```python
from build123d import *

# Parameters (mm, degrees)
EKSTR_ZYON_NCE1_DEPTH = 60
RADYUS1_R             = 10
KES_EKSTR_ZYON1_REACH = 236.137
IZIM2_R               = 4
IZIM2_R_2             = 2
KES_EKSTR_ZYON2_REACH = 234.491
IZIM3_R               = 2.5


with BuildPart() as part:
    # izim1 → Ekstr_zyon-_nce1 (new body)
    with BuildSketch(Plane.XY):
        Polygon((0, 0), (200, 0), (200, 90), (0, 90), (0, 94), (204, 94), (204, -4), (0, -4), align=None)
    extrude(amount=EKSTR_ZYON_NCE1_DEPTH)

    # Radyus1
    radyus1_edges = [part.edges().sort_by_distance(p)[0] for p in [
        (0, -2, 60),
        (0, 92, 60),
        (0, -2, 0),
        (0, 92, 0),
    ]]
    fillet(radyus1_edges, radius=RADYUS1_R)

    # izim2 → Kes-Ekstr_zyon1 (cut, up to next)
    with BuildSketch(Plane(origin=(0, 94, 0), x_dir=(1, 0, 0), z_dir=(0, 1, 0)), mode=Mode.PRIVATE) as kes_ekstr_zyon1_sk1:
        with Locations(Location((23, -30, 0), (0, 0, 270))):
            Circle(IZIM2_R)
    kes_ekstr_zyon1_tool1 = extrude(kes_ekstr_zyon1_sk1.sketch, amount=-KES_EKSTR_ZYON1_REACH, mode=Mode.PRIVATE) & part.part
    # izim2 → Kes-Ekstr_zyon1 (cut, up to next)
    with BuildSketch(Plane(origin=(0, 94, 0), x_dir=(1, 0, 0), z_dir=(0, 1, 0)), mode=Mode.PRIVATE) as kes_ekstr_zyon1_sk2:
        with Locations(Location((23, -22, 0), (0, 0, 270))):
            Circle(IZIM2_R_2)
    kes_ekstr_zyon1_tool2 = extrude(kes_ekstr_zyon1_sk2.sketch, amount=-KES_EKSTR_ZYON1_REACH, mode=Mode.PRIVATE) & part.part
    # izim2 → Kes-Ekstr_zyon1 (cut, up to next)
    with BuildSketch(Plane(origin=(0, 94, 0), x_dir=(1, 0, 0), z_dir=(0, 1, 0)), mode=Mode.PRIVATE) as kes_ekstr_zyon1_sk3:
        with Locations(Location((23, -38, 0), (0, 0, 270))):
            Circle(IZIM2_R_2)
    kes_ekstr_zyon1_tool3 = extrude(kes_ekstr_zyon1_sk3.sketch, amount=-KES_EKSTR_ZYON1_REACH, mode=Mode.PRIVATE) & part.part
    # izim2 → Kes-Ekstr_zyon1 (cut, up to next)
    with BuildSketch(Plane(origin=(0, 94, 0), x_dir=(1, 0, 0), z_dir=(0, 1, 0)), mode=Mode.PRIVATE) as kes_ekstr_zyon1_sk4:
        with Locations(Location((31, -30, 0), (0, 0, 270))):
            Circle(IZIM2_R_2)
    kes_ekstr_zyon1_tool4 = extrude(kes_ekstr_zyon1_sk4.sketch, amount=-KES_EKSTR_ZYON1_REACH, mode=Mode.PRIVATE) & part.part
    # izim2 → Kes-Ekstr_zyon1 (cut, up to next)
    with BuildSketch(Plane(origin=(0, 94, 0), x_dir=(1, 0, 0), z_dir=(0, 1, 0)), mode=Mode.PRIVATE) as kes_ekstr_zyon1_sk5:
        with Locations(Location((15, -30, 0), (0, 0, 270))):
            Circle(IZIM2_R_2)
    kes_ekstr_zyon1_tool5 = extrude(kes_ekstr_zyon1_sk5.sketch, amount=-KES_EKSTR_ZYON1_REACH, mode=Mode.PRIVATE) & part.part
    kes_ekstr_zyon1_1 = kes_ekstr_zyon1_tool1.solids().sort_by_distance((23, 94, 30))[0]
    add(kes_ekstr_zyon1_1, mode=Mode.SUBTRACT)
    kes_ekstr_zyon1_2 = kes_ekstr_zyon1_tool2.solids().sort_by_distance((23, 94, 22))[0]
    add(kes_ekstr_zyon1_2, mode=Mode.SUBTRACT)
    kes_ekstr_zyon1_3 = kes_ekstr_zyon1_tool3.solids().sort_by_distance((23, 94, 38))[0]
    add(kes_ekstr_zyon1_3, mode=Mode.SUBTRACT)
    kes_ekstr_zyon1_4 = kes_ekstr_zyon1_tool4.solids().sort_by_distance((31, 94, 30))[0]
    add(kes_ekstr_zyon1_4, mode=Mode.SUBTRACT)
    kes_ekstr_zyon1_5 = kes_ekstr_zyon1_tool5.solids().sort_by_distance((15, 94, 30))[0]
    add(kes_ekstr_zyon1_5, mode=Mode.SUBTRACT)
    kes_ekstr_zyon1 = kes_ekstr_zyon1_1 + kes_ekstr_zyon1_2 + kes_ekstr_zyon1_3 + kes_ekstr_zyon1_4 + kes_ekstr_zyon1_5  # Kes-Ekstr_zyon1 as one shape, for the pattern or mirror that repeats it

    # Aynalama1: Kes-Ekstr_zyon1 across plane
    add(kes_ekstr_zyon1.mirror(Plane.ZX.offset(45)), mode=Mode.SUBTRACT)

    # izim3 → Kes-Ekstr_zyon2 (cut, up to next)
    with BuildSketch(Plane(origin=(204, 0, 0), x_dir=(0, 0, -1), z_dir=(1, 0, 0)), mode=Mode.PRIVATE) as kes_ekstr_zyon2_sk1:
        with Locations((-30, 60)):
            Circle(IZIM3_R)
    kes_ekstr_zyon2_tool1 = extrude(kes_ekstr_zyon2_sk1.sketch, amount=-KES_EKSTR_ZYON2_REACH, mode=Mode.PRIVATE) & part.part
    # izim3 → Kes-Ekstr_zyon2 (cut, up to next)
    with BuildSketch(Plane(origin=(204, 0, 0), x_dir=(0, 0, -1), z_dir=(1, 0, 0)), mode=Mode.PRIVATE) as kes_ekstr_zyon2_sk2:
        with Locations(Location((-30, 30, 0), (0, 0, 180))):
            Circle(IZIM3_R)
    kes_ekstr_zyon2_tool2 = extrude(kes_ekstr_zyon2_sk2.sketch, amount=-KES_EKSTR_ZYON2_REACH, mode=Mode.PRIVATE) & part.part
    # izim3 → Kes-Ekstr_zyon2 (cut, up to next)
    with BuildSketch(Plane(origin=(204, 0, 0), x_dir=(0, 0, -1), z_dir=(1, 0, 0)), mode=Mode.PRIVATE) as kes_ekstr_zyon2_sk3:
        with Locations((-15, 45)):
            Circle(IZIM3_R)
    kes_ekstr_zyon2_tool3 = extrude(kes_ekstr_zyon2_sk3.sketch, amount=-KES_EKSTR_ZYON2_REACH, mode=Mode.PRIVATE) & part.part
    # izim3 → Kes-Ekstr_zyon2 (cut, up to next)
    with BuildSketch(Plane(origin=(204, 0, 0), x_dir=(0, 0, -1), z_dir=(1, 0, 0)), mode=Mode.PRIVATE) as kes_ekstr_zyon2_sk4:
        with Locations(Location((-45, 45, 0), (0, 0, 180))):
            Circle(IZIM3_R)
    kes_ekstr_zyon2_tool4 = extrude(kes_ekstr_zyon2_sk4.sketch, amount=-KES_EKSTR_ZYON2_REACH, mode=Mode.PRIVATE) & part.part
    add(kes_ekstr_zyon2_tool1.solids().sort_by_distance((204, 60, 30))[0], mode=Mode.SUBTRACT)
    add(kes_ekstr_zyon2_tool2.solids().sort_by_distance((204, 30, 30))[0], mode=Mode.SUBTRACT)
    add(kes_ekstr_zyon2_tool3.solids().sort_by_distance((204, 45, 15))[0], mode=Mode.SUBTRACT)
    add(kes_ekstr_zyon2_tool4.solids().sort_by_distance((204, 45, 45))[0], mode=Mode.SUBTRACT)


solid = part.part
```
Here's how the part is built. I have some questions about the finished solid (model axes, mm). A direction names the side the tool comes from. Give positions to 0.01 mm unless a question says otherwise; leave off trailing zeros. Loops run counter-clockwise (first coordinate to the right, second up) from the corner with the lowest first, then second, coordinate; pieces in that order, holes last. Notation, with made-up numbers: M -1,9 L 54,9 A26 ccw 54,39 Z; hole C -2.75,86 d8. An arc over 180 degrees is marked long. Use one line per item in the form item = value. Start each with the question number.
Q1. If we section it at C-C (y = 60): Write out the boundary of the cut face in (x, z).
Q2. I need wall thicknesses on line 1 along X through (y, z) = (91, 30); line 2 along Y through (x, z) = (176, 20); line 3 along Z through (x, y) = (201, 30). Which ranges of each line are inside material? Lowest first, please.
Q3. If we section it at D-D (x = 15): Write out the boundary of the cut face in (y, z).
Q4. If we section it at A-A (x = 147): Write out the boundary of the cut face in (y, z), then the cut area to 3 significant figures.
Q5. If we section it at B-B (z = 38): Write out the boundary of the cut face in (x, y), then the cut area to 3 significant figures.
Q6. Will these pins go through, and if not, where does the flat tip stop? pin 1 Ø10 at (y, z) = (76.5, 47.5) entering from -X; pin 2 Ø2.5 at (x, z) = (23, 38) entering from -Y; pin 3 Ø9 at (x, z) = (23, 30) entering from +Y.
Q7. Thinking about a two-plate mould opening in Z: for faces 3 (the flat face through (0, -2, 30)), 4 (the cylindrical face through (26.966, 92.028, 29.479)), 5 (the flat face through (136, -2, 60)), 6 (the cylindrical face through (202.03, 42.56, 15.54)), which applies, +Z half, -Z half, draft (parallel to the pull), parting line (faces both ways), or undercut?
Q8. Which directions (+Z, -Z, +X, -X, +Y, -Y) give clear straight access to the entire face, cutting with the end or side of a thin tool? Please do faces 1 (the flat face through (200, 44, 30)), 2 (the flat face through (136, -2, 0)).
Taken from the geometry:
q1.outline = M 200,0 L 204,0 L 204,27.5 L 200,27.5 Z; M 200,32.5 L 204,32.5 L 204,60 L 200,60 Z
q2.line_1 = 0 to 13, 17 to 19, 27 to 29, 33 to 204
q2.line_2 = -4 to 0, 90 to 94
q2.line_3 = 0 to 27.5, 32.5 to 60
q3.outline = M -4,0 L 0,0 L 0,28 L -4,28 Z; M -4,32 L 0,32 L 0,60 L -4,60 Z; M 90,0 L 94,0 L 94,28 L 90,28 Z; M 90,32 L 94,32 L 94,60 L 90,60 Z
q4.outline = M -4,0 L 0,0 L 0,60 L -4,60 Z; M 90,0 L 94,0 L 94,60 L 90,60 Z
q4.area = 480 mm^2
q5.outline = M 0,-4 L 21,-4 L 21,0 L 0,0 Z; M 0,90 L 21,90 L 21,94 L 0,94 Z; M 25,-4 L 204,-4 L 204,94 L 25,94 L 25,90 L 200,90 L 200,0 L 25,0 Z
q5.area = 1,960 mm^2
q6.pin_1 = 200
q6.pin_2 = through
q6.pin_3 = 94
q7.face_3 = draft
q7.face_4 = undercut
q7.face_5 = +Z half
q7.face_6 = undercut
q8.face_1 = +Z, -Z, -X
q8.face_2 = -Z, +X, -X, +Y, -Y
